Design review of the part built by this model. Coordinates are the model's own, in mm. A direction names the side the tool comes from. Round coordinates to 2 decimals unless told otherwise and drop trailing zeros. Write each loop counter-clockwise with the first axis right and the second up, starting at its lowest first coordinate (ties: lowest second). Pieces come first, ordered by that corner, then holes. Notation, with made-up numbers: M 4,53 L 34,53 A18 cw 34,88 Z; hole C -25,64.25 d4. An arc over 180 degrees is marked long. Use CSV: the item, a comma, the result in double quotes.
Autodesk Inventor part; units mm, degrees
ref_plane "Work Plane1" through (1.525, 0, 0) normal (0, 0, 1) x (1, 0, 0)
ref_plane "YZ Plane" through (0, 0, 0) normal (1, 0, 0) x (0, 1, 0)
ref_plane "XZ Plane" through (0, 0, 0) normal (0, 1, 0) x (-1, 0, 0)
sketch "Boceto1" plane through (0, 0, 0) normal (0, 0, 1) x (1, 0, 0)
  line L0 (0, 5.7) -> (0, 3.6617)
  line L1 (3.75, 4) -> (20, 4)
  line L2 (20, 4) -> (20, 0)
  line L3 (20, 0) -> (-0.6001, 0)
  line L4 (-0.7001, 0) -> (2.45, 0)
  line L5 (-0.6001, 0) -> (-0.6001, 5.7)
  line L6 (-0.6001, 5.7) -> (0, 5.7)
  line L7 (3.75, 4) -> (2.9831, 3.6617)
  line L8 (2.9831, 3.6617) -> (0, 3.6617)
  line L9 (0, -0.227) -> (0, 1.362)
  dimension "d0" = 20
  dimension "d1" = 16.25
  dimension "d2" = 8
  dimension "d9" = 0.6001
  dimension "d10" = 11.4
  dimension "d13" = 0.7669
  dimension "d14" = 7.3234
revolve "Cuerpo" add sketch "Boceto1" angle 360 about axis through (20, 0, 0) along (-1, 0, 0)
sketch "Boceto2" plane through (-0.6001, 0, 0) normal (-1, 0, 0) x (0, 0, 1)
  line L0 (0, 7.5056) -> (6.5, 3.7528)
  line L1 (6.5, 3.7528) -> (6.5, -3.7528)
  line L2 (6.5, -3.7528) -> (0, -7.5056)
  line L3 (0, -7.5056) -> (-6.5, -3.7528)
  line L4 (-6.5, -3.7528) -> (-6.5, 3.7528)
  line L5 (-6.5, 3.7528) -> (0, 7.5056)
  point P0 (0, 0)
  point P1 (0, 0)
  dimension "d11" = 13
extrude "Cabeza" add sketch "Boceto2" along normal blind 4.7
sketch "Boceto4" plane through (0, 0, 0) normal (0, 0, 1) x (1, 0, 0)
  line L0 (-5.3001, 6.5) -> (-5.3001, 7.5056)
  line L1 (-5.3001, 7.5056) -> (-4.7195, 7.5056)
  line L2 (-4.7195, 7.5056) -> (-5.3001, 6.5)
  line L3 (-1.2701, 0) -> (-0.0801, 0)
  line L4 (-0.6001, 7.5056) -> (-5.3001, 7.5056)
  line L5 (-5.3001, 3.7528) -> (-5.3001, 7.5056)
  dimension "d5" = 30
  dimension "d19" = 13
revolve "Chaflán1" cut sketch "Boceto4" angle 360 about axis through (-10, 0, 0) along (1, 0, 0)
thread "Rosca"
chamfer "Chaflán2" distance 0.7668 distance2 0.7669 1 edges at (20, -4, 0) measured on face at (20, 1.3194, 0.8842)
ref_plane "Work Plane1" through (1.525, 0, 0) normal (0, 0, 1) x (1, 0, 0)
equation "\"d0\" = NLG"
equation "\"d1\" = GEL"
equation "\"d2\" = GD"
equation "\"d10\" = SD2"
equation "\"d14\" = BDM"
equation "\"d11\" = SW"
equation "\"d3\" = KOH - SD"
equation "\"d5\" = ANG1"
equation "\"d19\" = SW0"
equation "\"d15\" = GEL"
equation "\"d6\" = -0.5 * SPD + 0.5 * GD"
equation "\"NLG\" = 20"
equation "\"GD\" = NND"
equation "\"BDM\" = 7.32342"
equation "\"KOH\" = 5.3"
equation "\"GEL\" = 16.25"
equation "\"SW\" = 13"
equation "\"SW0\" = 13"
equation "\"SPD\" = NND - 1.2269 * PTC"
equation "\"SD2\" = 11.4"
equation "\"SD\" = 0.6"
equation "\"ANG1\" = 30deg"
equation "\"GAL\" = 0.61345 * PTC"
equation "\"GUL\" = 0.61345 * PTC"
equation "\"RR\" = 0.4"
equation "\"GD1\" = THREADDIA - 1.2269 * PTC"
equation "\"THREADDIA\" = 8"
equation "\"TOA\" = 30deg"
equation "\"PTC\" = 1.25"
equation "\"NND\" = 8"
equation "\"E0\" = 1.155 * SW"
properties part number "DIN 933 - M8  x 20" material "Acero, suave"
1) The part is to be moulded in two halves that separate along X. For faces 4 (the face through (-5.2, 6.67, -0.15)), 5 (the face through (20, 0, 0)), 6 (the face through (-2.92, 5.66, 3.2)), 7 (the face through (1.47, -3.66, -0.16)), say which applies: released by +X, released by -X, zero draft, split by the parting line, or undercut.
Answers:
face 4,"released by -X"
face 5,"released by +X"
face 6,"zero draft"
face 7,"undercut"
2) Add section A-A on x = -2.5. Write out the cut boundary in (y, z), then the cut area to 3 significant figures.
Answers:
outline,"M -7.51,0 L -3.75,-6.5 L 3.75,-6.5 L 7.51,0 L 3.75,6.5 L -3.75,6.5 Z"
area,"146 mm²"
3) Machinability: for faces 1 (the face through (-5.2, -6.67, 0.15)), 2 (the face through (11.6, -0.867, -3.905)), 3 (the face through (0, 0, 4)), which of the approach directions +Z, -Z, +X, -X, +Y, -Y give a long, thin tool a straight path to every point of the face, cutting with its end or side? Answer none if there is none.
Answers:
face 1,"-X, -Y"
face 2,"+X"
face 3,"none"
4) Add section B-B on x = 5. Write out the cut boundary in (y, z).
Answers:
outline,"C 0,0 d8"
5) For pin 1 Ø5 at (y, z) = (-5.5, 4.5) entering from -X, flat-tipped, find the tip position at first contact; note if it passes through.
Answers:
pin 1,"x = -5.3"
6) Wall thickness on line 1 along X through (y, z) = (6, -1.75); line 2 along X through (y, z) = (3.25, -3.25); line 3 along Y through (x, z) = (5.25, -1.5): over which ranges is each line inside the solid? List them lowest first. Write a range as [from, to].
Answers:
line 1,"[-5.3, -0.6]"
line 2,"[-5.3, 0]"
line 3,"[-3.71, 3.71]"
